Verification items for the finished model (mm, model axes). A direction names the side the tool comes from. Round coordinates to 2 decimals unless told otherwise and drop trailing zeros. Write each loop counter-clockwise with the first axis right and the second up, starting at its lowest first coordinate (ties: lowest second). Pieces come first, ordered by that corner, then holes. Notation, with made-up numbers: (18, -6) - (39, -6) arc R13 ccw to (39, 4) - close; hole circle Ø9 at (36.25, 69.25). An arc over 180 degrees is marked (long way). Write each question's results on one line, items separated by ' | '.
```python
from build123d import *

# Parameters (mm, degrees)
F0_R     = 10
F1_DEPTH = 125
F2_R     = 50
F2_R_2   = 10
F3_DEPTH = 50
F5_DEPTH = 25


with BuildPart() as f1:
    # F0 (on Right) → F1 (new body)
    with BuildSketch(Plane.YZ):
        Circle(F0_R)
    extrude(amount=F1_DEPTH)

    # F2 (on face) → F3 (join)
    with BuildSketch(Plane.YZ.offset(125)):
        Circle(F2_R)
        Circle(F2_R_2, mode=Mode.SUBTRACT)
        Circle(F2_R_2)
    extrude(amount=F3_DEPTH)

    # F4 (on face) → F5 (join)
    with BuildSketch(Plane.YZ.offset(175)):
        with BuildLine():
            Line((-42.5, 42.5), (-42.5, 26.339134))
            ThreePointArc((-42.5, 26.339134), (-35.355339, 35.355339), (-26.339134, 42.5))
            Line((-26.339134, 42.5), (-42.5, 42.5))
        make_face()
        with BuildLine():
            ThreePointArc((26.339134, 42.5), (35.355339, 35.355339), (42.5, 26.339134))
            Line((42.5, 26.339134), (42.5, 42.5))
            Line((42.5, 42.5), (26.339134, 42.5))
        make_face()
        with BuildLine():
            Line((26.339134, -42.5), (42.5, -42.5))
            Line((42.5, -42.5), (42.5, -26.339134))
            ThreePointArc((42.5, -26.339134), (35.355339, -35.355339), (26.339134, -42.5))
        make_face()
        with BuildLine():
            Line((-42.5, -42.5), (-26.339134, -42.5))
            ThreePointArc((-26.339134, -42.5), (-35.355339, -35.355339), (-42.5, -26.339134))
            Line((-42.5, -26.339134), (-42.5, -42.5))
        make_face()
        with BuildLine():
            Line((-26.339134, -42.5), (26.339134, -42.5))
            ThreePointArc((26.339134, -42.5), (35.355339, -35.355339), (42.5, -26.339134))
            Line((42.5, -26.339134), (42.5, 26.339134))
            ThreePointArc((42.5, 26.339134), (35.355339, 35.355339), (26.339134, 42.5))
            Line((26.339134, 42.5), (-26.339134, 42.5))
            ThreePointArc((-26.339134, 42.5), (-35.355339, 35.355339), (-42.5, 26.339134))
            Line((-42.5, 26.339134), (-42.5, -26.339134))
            ThreePointArc((-42.5, -26.339134), (-35.355339, -35.355339), (-26.339134, -42.5))
        make_face()
    extrude(amount=-F5_DEPTH)

    # F6: F1 across face


with BuildPart() as f1_1:
    add(f1.part)
    add(f1.part.mirror(Plane.YZ.offset(175)))


solid = f1_1.part
```
(1) Section check A-A (y = 0). Record the cut outline in (x, z), plus the area to 3 significant figures.
Answer:
outline: (0, -10) - (125, -10) - (125, -50) - (225, -50) - (225, -10) - (350, -10) - (350, 10) - (225, 10) - (225, 50) - (125, 50) - (125, 10) - (0, 10) - close | area: 15,000 mm2
(2) Section check D-D (z = -14.5). Record the cut outline in (x, y).
Answer:
outline: (125, -47.85) - (225, -47.85) - (225, 47.85) - (125, 47.85) - close
(3) Set-up check for faces 1 (the flat face through (175, 42.5, 34)), 2 (the flat face through (175, -34, 42.5)), 3 (the cylindrical face through (288.38, -2.17, -9.76)): record each of +Z, -Z, +X, -X, +Y, -Y from which the full face is reachable in a straight line by a thin tool's end or side.
Answer:
face 1: +Z, +X, -X, +Y | face 2: +Z, +X, -X, -Y | face 3: +X
(4) Section check C-C (x = 115). Record the cut outline in (y, z), plus the area to 3 significant figures.
Answer:
outline: circle Ø20 at (0, 0) | area: 314 mm2
(5) Go/stop test with flat-tipped pins: pin 1 Ø8 at (y, z) = (33, -33) entering from -X; pin 2 Ø5 at (y, z) = (-31.5, 35.5) entering from +X; pin 3 Ø4 at (x, y) = (193.5, 6) entering from -Z. Record where each tip stops, or that it passes through.
Answer:
pin 1: x = 125 | pin 2: x = 225 | pin 3: z = -49.84
(6) Thickness scan on L1, parallel to X at y = 27, z = -41; L2, parallel to Z at x = 43.5, y = 0.5; L3, parallel to Z at x = 195, y = 1. Record the ranges inside material, lowest first.
Answer:
L1: 125 to 225 | L2: -9.99 to 9.99 | L3: -49.99 to 49.99
